Could you check a few things on this model? Use its own coordinates, in mm. Give positions to 0.01 mm unless a question says otherwise; leave off trailing zeros. Order: outer loops, then holes, each group sorted by start corner. A loop starts at its lowest first (then second) coordinate and runs counter-clockwise, first axis right, second up. Notation, with made-up numbers: (-5, 9.5) -> (22, 9.5) arc R25 cw to (22, 46.5) -> close; hole circle Ø8 at (26, 80). An arc over 180 degrees is marked (long way). One line per item, written item: value.
```python
from build123d import *

# Parameters (mm, degrees)
SKETCH1_W           = 150
SKETCH1_H           = 130
BOSS_EXTRUDE1_DEPTH = 3
CUT_EXTRUDE1_DEPTH  = 100.292497199


with BuildPart() as part:
    # Sketch1 → Boss-Extrude1 (new body)
    with BuildSketch(Plane(origin=(0, 0, 0), x_dir=(1, 0, 0), z_dir=(0, 1, 0))):
        Rectangle(SKETCH1_W, SKETCH1_H)
    extrude(amount=BOSS_EXTRUDE1_DEPTH)

    # Sketch2 → Cut-Extrude1 (cut, through all)
    with BuildSketch(Plane(origin=(0, 3, 0), x_dir=(1, 0, 0), z_dir=(0, 1, 0))):
        Polygon((-55, 65), (-75, 50), (-75, 65), align=None)
        Polygon((-75, -50), (-55, -65), (-75, -65), align=None)
        Polygon((75, -50), (55, -65), (75, -65), align=None)
        Polygon((55, 65), (75, 50), (75, 65), align=None)
    extrude(amount=-CUT_EXTRUDE1_DEPTH, mode=Mode.SUBTRACT)


solid = part.part
```
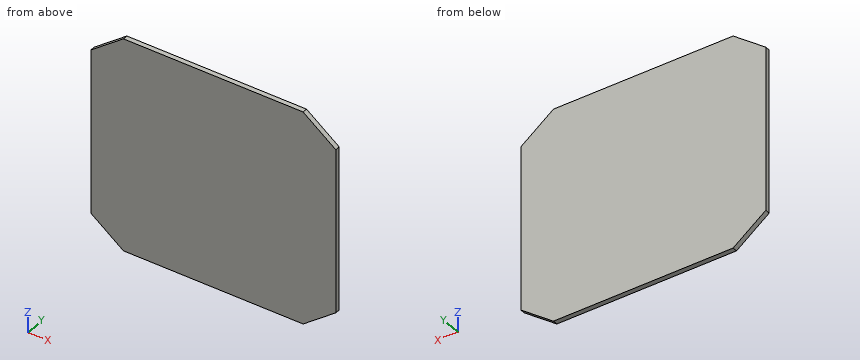
1) Suppose I cut it at A-A, the plane y = 1.8. Write out the boundary of the cut face in (x, z), then the cut area to 3 significant figures.
Answer below:
outline: (-75, -50) -> (-55, -65) -> (55, -65) -> (75, -50) -> (75, 50) -> (55, 65) -> (-55, 65) -> (-75, 50) -> close
area: 18,900 mm2
2) Suppose I cut it at B-B, the plane x = 62. Write out the boundary of the cut face in (y, z).
Answer below:
outline: (0, -59.75) -> (3, -59.75) -> (3, 59.75) -> (0, 59.75) -> close
3) If I drill on line 1 along X through (y, z) = (0.6, -53.5); line 2 along Z through (x, y) = (66.5, 0.6) (3 decimals); line 3 along X through (y, z) = (2, -50.5), over which ranges is the centre line in solid material (lowest first)?
Answer below:
line 1: x = -70.33 to 70.33
line 2: z = -56.375 to 56.375
line 3: x = -74.33 to 74.33
4) For P1, Ø6, axis at x = 10, z = 17, coming from the -Y side, with a flat end and sliding along its axis, tell me the tip position at first contact or that it passes through.
Answer below:
P1: stops at y = 0
